Could you check a few things on this model? Use its own coordinates, in mm. A direction names the side the tool comes from. Coordinates: 2 decimals unless noted, no trailing zeros. Write each loop counter-clockwise with the first axis right and the second up, starting at its lowest first coordinate (ties: lowest second). Pieces come first, ordered by that corner, then holes.
Item 1: Thinking about a two-plate mould opening in Y: for faces 3 (the cylindrical face through (12.724, 46.877, 0.507)), 4 (the flat face through (12, 38, 0)), which applies, +Y half, -Y half, draft (parallel to the pull), parting line (faces both ways), or undercut?
Item 2: Which directions (+Z, -Z, +X, -X, +Y, -Y) give clear straight access to the entire face, cutting with the end or side of a thin tool? Please do faces 1 (the cylindrical face through (12.721, 46.707, 0.507)), 2 (the flat face through (12, 38, 1)).
Item 3: For P1, Ø4, axis at x = 4.5, y = 35, coming from the -Z side, with a flat end and sliding along its axis, tell me the tip position at first contact or that it passes through.
Item 4: If I drill on probe 1 along X at (y, z) = (39.5, 0.25); probe 2 along Y at (x, z) = (7.5, 0.15); probe 3 along Y at (x, z) = (19.75, 0.4), over which ranges is the centre line in solid material (lowest first)?
Item 5: I want a section at A-A on y = 41.5. Please give me the cut outline in (x, z).
from build123d import *

# Parameters (mm, degrees)
PAD005_DEPTH      = 2
PAD005_DEPTH_BACK = 2
SKETCH021_W       = 25
SKETCH021_H       = 75
PAD020_DEPTH      = 1


with BuildPart() as body005:
    # Sketch006 → Pad005 (new body, two sides)
    with BuildSketch(Plane.XY) as pad005_sk:
        with BuildLine():
            ThreePointArc((21.884948, 37.50431), (12.518321, 46.87999), (3.125, 37.531055))
            Line((3.295001, 37.531055), (3.125, 37.531055))
            ThreePointArc((21.714948, 37.50431), (12.518321, 46.70999), (3.295001, 37.531055))
            Line((21.884948, 37.50431), (21.714948, 37.50431))
        make_face()
    extrude(amount=PAD005_DEPTH)
    extrude(pad005_sk.sketch, amount=-PAD005_DEPTH_BACK)


with BuildPart() as body019:
    # Sketch021 → Pad020 (new body)
    with BuildSketch(Plane.XY):
        with Locations((12.5, 37.5)):
            Rectangle(SKETCH021_W, SKETCH021_H)
    extrude(amount=PAD020_DEPTH)

    # Boolean004: cut Body005
    add(body005.part, mode=Mode.SUBTRACT)


solid = body019.part
Response values:
1. face 3: undercut
1. face 4: draft
2. face 1: +Z, -Z
2. face 2: +Z, +X, -X, +Y, -Y
3. P1: stops at z = 0
4. probe 1: x = 0 to 3.34, 3.51 to 21.5, 21.67 to 25
4. probe 2: y = 0 to 45.23, 45.43 to 75
4. probe 3: y = 0 to 43.19, 43.46 to 75
5. outline: (0, 0) - (4.02, 0) - (4.02, 1) - (0, 1) - close; (4.21, 0) - (20.8, 0) - (20.8, 1) - (4.21, 1) - close; (20.99, 0) - (25, 0) - (25, 1) - (20.99, 1) - close
